from build123d import *

# Parameters (mm, degrees)
SKETCH_1_W                   = 26
SKETCH_1_H                   = 15
EXTRUDE_1_DEPTH              = 5
SKETCH_2_W                   = 26
SKETCH_2_H                   = 15
EXTRUDE_2_DEPTH              = 1
HOLE_WIZARD_M3_1_AT_2_COUNT  = 2
HOLE_WIZARD_M3_1_AT_2_PITCH  = 6
HOLE_WIZARD_M3_2_D           = 2.5
HOLE_WIZARD_M3_2_DEPTH       = 7
HOLE_WIZARD_M3_2_TIP         = 0.751075774
HOLE_WIZARD_M3_3_D           = 2.5
HOLE_WIZARD_M3_3_CSINK_D     = 3.05
HOLE_WIZARD_M3_3_CSINK_ANGLE = 90


with BuildPart() as part:
    # 草图1 → 凸台-拉伸1 (new body)
    with BuildSketch(Plane.XY):
        Rectangle(SKETCH_1_W, SKETCH_1_H)
    extrude(amount=EXTRUDE_1_DEPTH)

    # 草图2 → 凸台-拉伸2 (add)
    with BuildSketch(Plane.XY.offset(5)):
        Rectangle(SKETCH_2_W, SKETCH_2_H)
    extrude(amount=EXTRUDE_2_DEPTH)

    # 草图4 → M3 螺纹孔1 (revolve, cut)
    with BuildSketch(Plane(origin=(-13, -3, 3), x_dir=(0, 0, 1), z_dir=(0, 1, 0))):
        Polygon((0, 0), (0, 5.751075774), (1.25, 5), (1.25, 0), align=None)
    hole_wizard_m3_1 = revolve(axis=Axis((-19.35, -3, 3), (1, 0, 0)), mode=Mode.SUBTRACT)

    # M3 螺纹孔1 at 2: M3 螺纹孔1 ×2
    with Locations(*[(0, i * HOLE_WIZARD_M3_1_AT_2_PITCH, 0) for i in range(1, HOLE_WIZARD_M3_1_AT_2_COUNT)]):
        add(hole_wizard_m3_1, mode=Mode.SUBTRACT)

    # 镜向1: M3 螺纹孔1 across plane
    add(hole_wizard_m3_1.mirror(Plane(origin=(0, 0, 0), x_dir=(0, 0, 1), z_dir=(1, 0, 0))), mode=Mode.SUBTRACT)

    # 镜向1 copy 1 sketch → 镜向1 copy 1 (revolve, cut)
    with BuildSketch(Plane(origin=(13, 3, 3), x_dir=(0, 0, 1), z_dir=(0, 1, 0))):
        Polygon((0, 0), (0, -5.751075774), (1.25, -5), (1.25, 0), align=None)
    revolve(axis=Axis((19.35, 3, 3), (1, 0, 0)), mode=Mode.SUBTRACT)

    # M3 螺纹孔2
    with Locations(Plane(origin=(-5, 7.5, 3), x_dir=(0, 0, 1), z_dir=(0, 1, 0))):
        with Locations((0, 0), (0, 10)):
            Hole(HOLE_WIZARD_M3_2_D / 2, depth=HOLE_WIZARD_M3_2_DEPTH)
            with Locations((0, 0, -(HOLE_WIZARD_M3_2_DEPTH + HOLE_WIZARD_M3_2_TIP / 2))):  # 118° drill point
                Cone(0, HOLE_WIZARD_M3_2_D / 2, HOLE_WIZARD_M3_2_TIP, mode=Mode.SUBTRACT)

    # M3 螺纹孔3 (through all)
    with Locations(Plane.XY.offset(6)):
        with Locations((8, 0)):
            CounterSinkHole(HOLE_WIZARD_M3_3_D / 2, HOLE_WIZARD_M3_3_CSINK_D / 2, counter_sink_angle=HOLE_WIZARD_M3_3_CSINK_ANGLE)


solid = part.part
Here's how the part is built. I have some questions about the finished solid (model axes, mm). A direction names the side the tool comes from. Round coordinates to 2 decimals unless told otherwise and drop trailing zeros. Loops run counter-clockwise (first coordinate to the right, second up) from the corner with the lowest first, then second, coordinate; pieces in that order, holes last.
1. We'd pull the mould along Z, two halves only. Please class faces 5 (the face through (-10.54, 2.62, 4.19)), 6 (the face through (9.25, 0.05, 2.82)), 7 (the face through (0, 0, 6)): +Z half, -Z half, draft (parallel to the pull), parting line (faces both ways), or undercut.
Answer list:
face 5: undercut
face 6: draft
face 7: +Z half
2. If we section it at C-C on x = 9: Count the separate pieces of the cut face and the enclosed holes in it, plus the area to 3 significant figures.
Answer list:
separate pieces: 2
enclosed holes: 2
area: 71.1 mm2
3. Which directions (+Z, -Z, +X, -X, +Y, -Y) give clear straight access to the entire face, cutting with the end or side of a thin tool? Please do faces 1 (the face through (3.891, 3.951, 2.423)), 2 (the face through (0, 0, 0)), 3 (the face through (-10.54, -3.38, 4.19)), 4 (the face through (10.54, -3.38, 4.19)).
Answer list:
face 1: +Y
face 2: -Z, +X, -X, +Y, -Y
face 3: -X
face 4: +X
4. If I drill on line 1 along Y through (x, z) = (-11, 3); line 2 along X through (y, z) = (3.75, 3.9); line 3 along Z through (x, y) = (5, 3.25), over which ranges is the centre line in solid material (lowest first)?
Answer list:
line 1: y = -7.5 to -4.25, -1.75 to 1.75, 4.25 to 7.5
line 2: x = -7.95 to -5.87, -4.13 to 4.13, 5.87 to 7.95
line 3: z = 0 to 1.75, 4.25 to 6
5. If we section it at B-B on y = 6.5: Write out the boundary of the cut face in (x, z).
Answer list:
outline: (-13, 0) - (13, 0) - (13, 6) - (-13, 6) - close; hole circle Ø2.5 at (-5, 3); hole circle Ø2.5 at (5, 3)
6. If we section it at A-A on y = 0: Write out the boundary of the cut face in (x, z) (3 decimals).
Answer list:
outline: (-13, 0) - (6.75, 0) - (6.75, 5.725) - (6.475, 6) - (-13, 6) - close; (9.25, 0) - (13, 0) - (13, 6) - (9.525, 6) - (9.25, 5.725) - close; hole circle Ø0.836 at (-5, 3); hole circle Ø0.836 at (5, 3)
